```python
from build123d import *

# Parameters (mm, degrees)
SKETCH1_W               = 8
SKETCH1_H               = 8
BOSS_EXTRUDE1_DEPTH     = 3
CUT_EXTRUDE1_DEPTH      = 12.704699911
CUT_EXTRUDE1_DEPTH_BACK = 12.704699911
CUT_EXTRUDE2_DEPTH      = 11
SKETCH4_R               = 1.8
CUT_EXTRUDE3_DEPTH      = 0.8
SKETCH5_W               = 8
SKETCH5_H               = 1
BOSS_EXTRUDE2_DEPTH     = 2
FILLET1_R               = 4
CUT_EXTRUDE4_DEPTH      = 0.4
CUT_EXTRUDE5_DEPTH      = 0.4


with BuildPart() as part:
    # Sketch1 → Boss-Extrude1 (new body)
    with BuildSketch(Plane(origin=(0, 0, 0), x_dir=(1, 0, 0), z_dir=(0, 1, 0))):
        with Locations((4, 4)):
            Rectangle(SKETCH1_W, SKETCH1_H)
    extrude(amount=BOSS_EXTRUDE1_DEPTH)

    # Sketch2 → Cut-Extrude1 (cut, two sides: drawn at the far end of the back side and taken through both)
    with BuildSketch(Plane.XY.offset(-CUT_EXTRUDE1_DEPTH_BACK)):
        Polygon((0, 0), (0.6, 3), (0, 3), align=None)
        Polygon((8, 0), (7.4, 3), (8, 3), align=None)
    extrude(amount=CUT_EXTRUDE1_DEPTH + CUT_EXTRUDE1_DEPTH_BACK, mode=Mode.SUBTRACT)

    # Sketch3 → Cut-Extrude2 (cut)
    with BuildSketch(Plane(origin=(0, 0, 0), x_dir=(0, 0, -1), z_dir=(1, 0, 0))):
        Polygon((0, 0), (0.6, 3), (0, 3), align=None)
        Polygon((8, 3), (7.4, 3), (8, 0), align=None)
    extrude(amount=CUT_EXTRUDE2_DEPTH, mode=Mode.SUBTRACT)

    # Sketch4 → Cut-Extrude3 (cut)
    with BuildSketch(Plane.XZ):
        with Locations(Location((4, -3.75, 0), (0, 0, 270))):
            Circle(SKETCH4_R)
    extrude(amount=-CUT_EXTRUDE3_DEPTH, mode=Mode.SUBTRACT)

    # Sketch5 → Boss-Extrude2 (add)
    with BuildSketch(Plane.XZ):
        with Locations((4, -7.5)):
            Rectangle(SKETCH5_W, SKETCH5_H)
    extrude(amount=BOSS_EXTRUDE2_DEPTH)

    # Fillet1
    # the kernel refuses this fillet: 4 mm, written as the material it takes off along each edge
    with BuildSketch(Plane(origin=(8, -2, -16.660254038), x_dir=(0, 1, 0), z_dir=(0, 0, 1)), Plane(origin=(0, -2, 1.660254038), x_dir=(0, 1, 0), z_dir=(0, 0, -1))) as fillet1_piece_1:
        with BuildLine():
            CenterArc((4, 3.464101615), FILLET1_R, 180, 60)
            Line((0, 3.464101615), (-0.08, 3.464101615))
            Line((-0.08, 3.464101615), (-0.08, 0))
            Line((-0.08, 0), (0, -0.08))
            ThreePointArc((0, -0.08), (1, -0.08), (1.96, -0.069282032))
            Line((1.96, -0.069282032), (2, 0))
        make_face()
    extrude(amount=18.320508076, mode=Mode.SUBTRACT)

    # Sketch6 → Cut-Extrude4 (cut)
    with BuildSketch(Plane(origin=(0, 3, 0), x_dir=(1, 0, 0), z_dir=(0, 1, 0))):
        Polygon((2.358967796, 2.025988971), (1.401435745, 6.025988971), (2.189897284, 6.025988971), (2.811692155, 3.278392817), (3.469544719, 6.025988971), (4.519224207, 6.025988971), (5.170666514, 3.231918458), (5.790858822, 6.025988971), (6.580922925, 6.025988971), (5.641019078, 2.025988971), (4.688294719, 2.025988971), (3.991179335, 5.016373586), (3.275634463, 2.025988971), align=None)
    extrude(amount=-CUT_EXTRUDE4_DEPTH, mode=Mode.SUBTRACT)

    # Sketch7 → Cut-Extrude5 (cut)
    with BuildSketch(Plane(origin=(0, 3, 0), x_dir=(1, 0, 0), z_dir=(0, 1, 0))):
        with BuildLine():
            Line((7.025079926, 1.261869909), (7.025079926, 0.954177602))
            Line((7.025079926, 0.954177602), (5.978926079, 0.954177602))
            add(Edge.make_bspline(
                [(5.978926079, 0.954177602), (5.982468114, 0.980474374), (5.989550197, 1.033053173), (6.011445466, 1.109857564), (6.040668149, 1.184805528), (6.072383822, 1.245794978), (6.103928572, 1.294889387), (6.132549124, 1.335117725), (6.166692393, 1.37791895), (6.205862922, 1.423638586), (6.249844239, 1.472419552), (6.298964472, 1.524080492), (6.353457933, 1.578374089), (6.391795053, 1.615242112), (6.411618387, 1.634305807)],
                knots=[0, 0, 0, 0, 1.156289446, 2.311930546, 3.473459201, 4.661751613, 5.303057008, 6.018253237, 6.81459331, 7.690699809, 8.644447906, 9.679642995, 10.800191253, 12, 12, 12, 12], degree=3))
            add(Edge.make_bspline(
                [(6.411618387, 1.634305807), (6.427437635, 1.649575712), (6.457552822, 1.678645113), (6.500436909, 1.720271317), (6.538136439, 1.758537631), (6.571439659, 1.79245241), (6.599577217, 1.822879209), (6.622919237, 1.849340182), (6.641761343, 1.871943086), (6.651966244, 1.886282382), (6.656490182, 1.89263914)],
                knots=[0, 0, 0, 0, 1.480720495, 2.818855715, 4.024636094, 5.098235712, 6.019786162, 6.815086302, 7.474715479, 8, 8, 8, 8], degree=3))
            add(Edge.make_bspline(
                [(6.656490182, 1.89263914), (6.665754103, 1.908027503), (6.683623134, 1.937709873), (6.703218009, 1.984385935), (6.714979583, 2.031052356), (6.71659359, 2.062234592), (6.717387618, 2.077575038)],
                knots=[0, 0, 0, 0, 1.0911822, 2.104764037, 3.067617678, 4, 4, 4, 4], degree=3))
            add(Edge.make_bspline(
                [(6.717387618, 2.077575038), (6.716811351, 2.093538834), (6.7157211, 2.123741092), (6.706579153, 2.166362064), (6.690367393, 2.203000826), (6.668046783, 2.233769843), (6.639822327, 2.257877251), (6.606827118, 2.275690284), (6.568578157, 2.285538571), (6.541694532, 2.286833928), (6.527644028, 2.287510935)],
                knots=[0, 0, 0, 0, 1.193122327, 2.257294386, 3.237245624, 4.168877528, 5.075331632, 5.990371598, 6.949684428, 8, 8, 8, 8], degree=3))
            add(Edge.make_bspline(
                [(6.527644028, 2.287510935), (6.513688449, 2.286878661), (6.486729282, 2.285657243), (6.448414457, 2.274987105), (6.414896057, 2.256515974), (6.391009062, 2.235466338), (6.374872264, 2.214997095), (6.363877213, 2.197159499), (6.354400337, 2.17689052), (6.346003035, 2.154418352), (6.339370115, 2.129485554), (6.334028373, 2.102282013), (6.329723702, 2.072661336), (6.328354741, 2.052055079), (6.327644028, 2.041357089)],
                knots=[0, 0, 0, 0, 1.402788338, 2.709884207, 3.961032948, 5.225417836, 5.883680772, 6.578928686, 7.329201998, 8.132101139, 8.990263233, 9.922304639, 10.921339128, 12, 12, 12, 12], degree=3))
            Line((6.327644028, 2.041357089), (6.01995172, 2.071485294))
            add(Edge.make_bspline(
                [(6.01995172, 2.071485294), (6.022425519, 2.092258403), (6.027221819, 2.132534142), (6.039191066, 2.190383991), (6.054349674, 2.243753088), (6.073420305, 2.292542389), (6.095614746, 2.337062147), (6.122065099, 2.376644317), (6.15184716, 2.411727355), (6.184986668, 2.44229259), (6.221272944, 2.468437258), (6.259348879, 2.491775386), (6.299958585, 2.510920071), (6.342654946, 2.526698167), (6.387418668, 2.539307895), (6.434456788, 2.547645276), (6.483479006, 2.553509822), (6.516941776, 2.553951654), (6.534054285, 2.554177602)],
                knots=[0, 0, 0, 0, 1.270971563, 2.464210789, 3.586263665, 4.638946707, 5.643716971, 6.603612468, 7.52484387, 8.434700188, 9.336036235, 10.239171475, 11.145359471, 12.059630629, 13.003312604, 13.96741569, 14.960557767, 16, 16, 16, 16], degree=3))
            add(Edge.make_bspline(
                [(6.534054285, 2.554177602), (6.552657792, 2.553820052), (6.58889046, 2.553123679), (6.641783721, 2.547373025), (6.69147314, 2.537345926), (6.738393137, 2.524063615), (6.782061867, 2.506330758), (6.82284322, 2.484892472), (6.860095371, 2.458935129), (6.894373612, 2.429874295), (6.925015616, 2.397916799), (6.95185524, 2.363828728), (6.974341388, 2.327633829), (6.993210719, 2.289773279), (7.007221071, 2.249637846), (7.017429622, 2.207782494), (7.024198302, 2.164011958), (7.024782801, 2.134117674), (7.025079926, 2.118921192)],
                knots=[0, 0, 0, 0, 1.210756838, 2.35810096, 3.457354827, 4.507168606, 5.527358126, 6.519769748, 7.499700793, 8.476517721, 9.440526811, 10.376769937, 11.295256217, 12.209626307, 13.124630862, 14.055668209, 15.011616881, 16, 16, 16, 16], degree=3))
            add(Edge.make_bspline(
                [(7.025079926, 2.118921192), (7.024688468, 2.101480457), (7.023911876, 2.066880717), (7.016476584, 2.015731964), (7.005116907, 1.965762694), (6.988328197, 1.916850789), (6.967047205, 1.867822963), (6.939615495, 1.818569171), (6.907765206, 1.767604004), (6.882827684, 1.7346528), (6.86995172, 1.71763914)],
                knots=[0, 0, 0, 0, 0.953409949, 1.89141903, 2.821310783, 3.752688675, 4.715703262, 5.740811754, 6.833515735, 8, 8, 8, 8], degree=3))
            add(Edge.make_bspline(
                [(6.86995172, 1.71763914), (6.865085171, 1.711509707), (6.854662151, 1.698381883), (6.836929855, 1.678252394), (6.816379649, 1.656264646), (6.793301796, 1.632007081), (6.766933989, 1.606338723), (6.738224942, 1.578186143), (6.705911376, 1.548989439), (6.672442351, 1.518020294), (6.638827847, 1.487878461), (6.607931272, 1.459250402), (6.579866901, 1.433920718), (6.555941744, 1.410491095), (6.534748531, 1.390560588), (6.517051134, 1.373107183), (6.502518393, 1.358553413), (6.482493212, 1.335867777), (6.457013442, 1.305185447), (6.439087381, 1.275867612), (6.430528644, 1.261869909)],
                knots=[0, 0, 0, 0, 0.665555651, 1.425465941, 2.280616993, 3.225313414, 4.272635571, 5.410053715, 6.644756443, 7.976022804, 9.288331007, 10.484517221, 11.558462543, 12.503158964, 13.33222979, 14.032602617, 14.617328242, 15.080653724, 16.606167857, 18, 18, 18, 18], degree=3))
            Line((6.430528644, 1.261869909), (7.025079926, 1.261869909))
        make_face()
    extrude(amount=-CUT_EXTRUDE5_DEPTH, mode=Mode.SUBTRACT)


solid = part.part
```
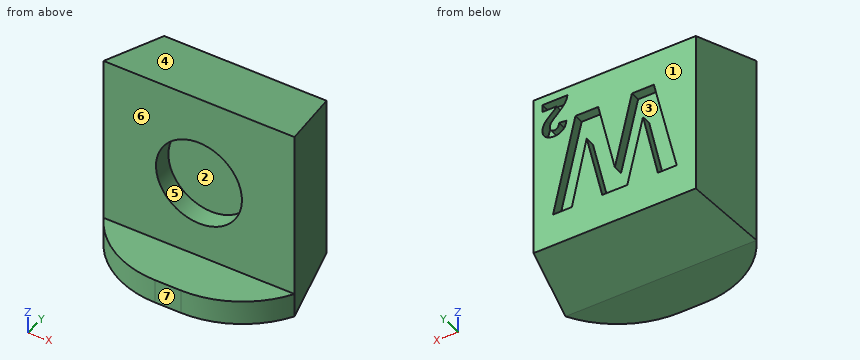
The model under review builds one solid part; all positions refer to its coordinate system, in mm. Face numbers are marked on the shaded views. A direction names the side the tool comes from. Coordinates: 2 decimals unless noted, no trailing zeros. Order: outer loops, then holes, each group sorted by start corner. A loop starts at its lowest first (then second) coordinate and runs counter-clockwise, first axis right, second up. Notation, with made-up numbers: (5.25, 38) -> (59.25, 38) arc R21 cw to (59.25, 68) -> close; hole circle Ø2 at (89, 75). An arc over 180 degrees is marked (long way). Answer in a Markdown table with one row per item. Add a question column.
Item 1: We need section C-C on x = 2.5. Write out the cut boundary in (y, z).
Item 2: Clearance check with flat-ended pins moving along their axes: pin 1 (1 mm diameter, centred on x = 5, y = -1, fed in from +Z); pin 2 (3 mm diameter, centred on y = 0.5, z = -2.5, fed in from +X); pin 3 (1.1 mm diameter, centred on x = 3.5, z = -4.5, fed in from -Y); pin 4 (4 mm diameter, centred on x = 4, z = -3.75, fed in from -Y). State where each tip first meets the part, or that it passes through.
Item 3: We need section D-D on y = 1.25. Write out the cut boundary in (x, z), plus the area to 4 significant figures.
Item 4: Machinability: for the marked faces 5, 6 and 7, which of the approach directions +Z, -Z, +X, -X, +Y, -Y give a long, thin tool a straight path to every point of the face, cutting with its end or side? Answer none if there is none.
Item 5: We need section B-B on z = -3.5. Write out the cut boundary in (x, y), plus the area to 3 significant figures.
Item 6: We need section A-A on y = 0.1. Write out the cut boundary in (x, z).
Item 7: To check wall thickness, follow probe 1 along Y at (x, z) = (5, -2.5); probe 2 along Y at (x, z) = (4, -5.75); probe 3 along Z at (x, y) = (4, -0.75). State the ranges of each line that lie inside material, in increasing order.
Item 8: Mouldability with a two-part tool opening along Z and no side actions: class the marked faces 1, 2, 3 and 4 as +Z half, -Z half, draft (parallel to the pull), parting line (faces both ways), or undercut.
Final values:
| question | item | result |
|---|---|---|
| 1 | outline | (-1.88, -8) -> (0, -8) -> (3, -7.4) -> (3, -4.66) -> (2.6, -4.66) -> (2.6, -2.03) -> (3, -2.03) -> (3, -0.6) -> (0, 0) -> (0, -2.76) -> (0.8, -2.76) -> (0.8, -4.74) -> (0, -4.74) -> (0, -7) -> (-1.88, -7) -> close |
| 2 | pin 1 | stops at z = -7 |
| 2 | pin 2 | stops at x = 8 |
| 2 | pin 3 | stops at y = 0.8 |
| 2 | pin 4 | stops at y = 0 |
| 3 | outline | (0.25, -7.75) -> (7.75, -7.75) -> (7.75, -0.25) -> (0.25, -0.25) -> close |
| 3 | area | 56.25 mm2 |
| 4 | face 5 | -Y |
| 4 | face 6 | +Z, +X, -X, -Y |
| 4 | face 7 | +Z, -Z, +X, -X, -Y |
| 5 | outline | (0, 0) -> (2.22, 0) -> (2.22, 0.8) -> (5.78, 0.8) -> (5.78, 0) -> (8, 0) -> (7.4, 3) -> (5.99, 3) -> (5.99, 2.6) -> (5.23, 2.6) -> (5.23, 3) -> (5.11, 3) -> (5.11, 2.6) -> (4.34, 2.6) -> (4.34, 3) -> (3.63, 3) -> (3.63, 2.6) -> (2.86, 2.6) -> (2.86, 3) -> (2.76, 3) -> (2.76, 2.6) -> (2.01, 2.6) -> (2.01, 3) -> (0.6, 3) -> close |
| 5 | area | 18.1 mm2 |
| 6 | outline | (0.02, -7.98) -> (7.98, -7.98) -> (7.98, -0.02) -> (0.02, -0.02) -> close; hole circle Ø3.6 at (4, -3.75) |
| 7 | probe 1 | y = 0.8 to 2.6 |
| 7 | probe 2 | y = 0 to 2.6 |
| 7 | probe 3 | z = -8 to -7 |
| 8 | face 1 | draft |
| 8 | face 2 | undercut |
| 8 | face 3 | undercut |
| 8 | face 4 | +Z half |
